The model under review builds one solid part; all positions refer to its coordinate system, in mm. A direction names the side the tool comes from. Round coordinates to 2 decimals unless told otherwise and drop trailing zeros. Loops run counter-clockwise (first coordinate to the right, second up) from the corner with the lowest first, then second, coordinate; pieces in that order, holes last. Notation, with made-up numbers: M 31,65 L 63,65 A9 cw 63,71 Z; hole C 50,89 d5. An arc over 180 degrees is marked long. Return JSON: item names as keys, results as strings. Group by question number.
Q1. Consider section D-D (x = -7). State the section outline as (y, z) points (3 decimals), and give its area (3 significant figures).
Q2. Consider section C-C (y = -1). State the section outline as (x, z) points, and give its area (3 significant figures).
Q3. Draft analysis for pull direction X (two halves, no side actions). For faces 1 (the face through (-12.5, 0, -17)), 2 (the face through (20, 0, 0)), 3 (the face through (10.577, -0.042, 10.636)), state which applies: pulls with the +X half, pulls with the -X half, needs draft (parallel to the pull), parting line crosses it, or undercut.
Q4. To check wall thickness, follow line 1 along Z through (x, y) = (-18, -2.5); line 2 along X through (y, z) = (-15, 6); line 3 along X through (y, z) = (-10, -5.5). State the ranges of each line that lie inside material, in increasing order.
Q5. Clearance check with flat-ended pins moving along their axes: pin 1 Ø2.5 at (x, y) = (17, 3) entering from +Z; pin 2 Ø1.5 at (x, z) = (10, 4.5) entering from +Y; pin 3 Ø1.5 at (x, y) = (7, 1) entering from +Z; pin 4 Ø6 at (y, z) = (-1, -15) entering from -X. State where each tip first meets the part, or that it passes through.
Q6. For faces 4 (the face through (17, 0, 12.5)), 5 (the face through (12.5, 0, -17)), 6 (the face through (-17, 0, 12.5)), list the 3-axis set-ups (+Z, -Z, +X, -X, +Y, -Y) from which the entire face can be reached by the end or side of a thin tool; tool diameter is ignored.
Q7. Consider section A-A (y = -12.5). State the section outline as (x, z) points.
Q8. Consider section B-B (z = -11). Count the separate pieces of the cut face and the enclosed holes in it, and give its area (3 significant figures).
from build123d import *
from OCP.BRepAlgoAPI import BRepAlgoAPI_Cut
from OCP.TopTools import TopTools_ListOfShape

# Parameters (mm, degrees)
CUT_EXTRUDE_2_DEPTH      = 59.108987417
CUT_EXTRUDE_2_DEPTH_BACK = 59.108987417
SKETCH_6_W               = 109.700764472
SKETCH_6_H               = 102.082655829
SKETCH_6_W_2             = 40
SKETCH_6_H_2             = 40
SKETCH_7_W               = 10.430230832
SKETCH_7_H               = 9.900213331
CUT_EXTRUDE_3_DEPTH      = 66.9796091
SKETCH_8_W               = 20.261670598
SKETCH_8_H               = 3
SKETCH_9_W               = 20.800473715
SKETCH_9_H               = 3
SKETCH_11_W              = 20.381404624
SKETCH_11_H              = 3
SKETCH_12_W              = 21.399143843
SKETCH_12_H              = 3


with BuildPart() as part:
    # Sketch 3 → Revolve 1 (revolve)
    with BuildSketch(Plane(origin=(0, 0, 0), x_dir=(0, 0, -1), z_dir=(1, 0, 0))):
        with BuildLine():
            Line((0, 40), (0, -40))
            ThreePointArc((0, -40), (40, 0), (0, 40))
        make_face()
    revolve(axis=Axis((0, 40, 0), (0, -1, 0)))

    # Sketch 4 → Cut-Revolve 3 (revolve, cut)
    with BuildSketch(Plane.XY, mode=Mode.PRIVATE) as cut_revolve_3_sk:
        Polygon((-25, 50), (25, 50), (12.5, 20), (-12.5, 20), align=None)
    revolve(cut_revolve_3_sk.sketch.rotate(Axis((-55.247864245, 0, 0), (1, 0, 0)), 90), axis=Axis((-55.247864245, 0, 0), (1, 0, 0)), mode=Mode.SUBTRACT)


with BuildPart() as cut_revolve_4_tool:
    # Sketch 5 → Cut-Revolve 4 (revolve)
    with BuildSketch(Plane(origin=(0, 0, 0), x_dir=(1, 0, 0), z_dir=(0, 1, 0))):
        Polygon((-50, 25), (-50, -25), (-20, -12.5), (-20, 12.5), align=None)
    revolve(axis=Axis((0, 0, -44.002313129), (0, 0, 1)))


with BuildPart() as part_1:
    add(part.part)

    # Cut-Revolve 4: cut by cut_revolve_4_tool, with a tolerance
    cut_revolve_4_stock = TopTools_ListOfShape()
    cut_revolve_4_stock.Append(part_1.part.wrapped)
    cut_revolve_4_tools = TopTools_ListOfShape()
    cut_revolve_4_tools.Append(cut_revolve_4_tool.part.wrapped)
    cut_revolve_4_cut = BRepAlgoAPI_Cut()
    cut_revolve_4_cut.SetArguments(cut_revolve_4_stock)
    cut_revolve_4_cut.SetTools(cut_revolve_4_tools)
    cut_revolve_4_cut.SetFuzzyValue(0.00001)
    cut_revolve_4_cut.Build()
    add(Compound.cast(cut_revolve_4_cut.Shape()).solids(), mode=Mode.REPLACE)

    # Sketch 6 → Cut-Extrude 2 (cut, two sides: drawn at the far end of the back side and taken through both)
    with BuildSketch(Plane(origin=(0, 0, 0), x_dir=(1, 0, 0), z_dir=(0, 1, 0)).offset(-CUT_EXTRUDE_2_DEPTH_BACK)):
        with Locations((-5.024851986, -5.217653308)):
            Rectangle(SKETCH_6_W, SKETCH_6_H)
        Rectangle(SKETCH_6_W_2, SKETCH_6_H_2, mode=Mode.SUBTRACT)
    extrude(amount=CUT_EXTRUDE_2_DEPTH + CUT_EXTRUDE_2_DEPTH_BACK, mode=Mode.SUBTRACT)

    # Sketch 7 → Cut-Extrude 3 (cut, through all)
    with BuildSketch(Plane(origin=(0, 29.80481839, 0), x_dir=(1, 0, 0), z_dir=(0, 1, 0))):
        Polygon((-12.5, 20), (-12.5, 12.5), (-20, 12.5), (-20, 22.400213331), (-12.5, 22.400213331), align=None)
        with Locations((17.715115416, 17.450106666)):
            Rectangle(SKETCH_7_W, SKETCH_7_H)
        Polygon((-12.5, -12.5), (-12.5, -22.2886307), (-23.264978728, -21.674926225), (-21.87019583, -13.864142), (-20, -12.5), align=None)
        Polygon((12.5, -12.5), (12.5, -20), (16.291064241, -21.981778462), (20, -20), (23.264978728, -15.681813192), (21.632489364, -12.626578567), (20, -12.5), align=None)
    extrude(amount=-CUT_EXTRUDE_3_DEPTH, mode=Mode.SUBTRACT)

    # Sketch 8 → Cut-Revolve 5 (revolve, cut)
    with BuildSketch(Plane(origin=(0, 0, 0), x_dir=(-0.7071067811865477, 0, -0.7071067811865475), z_dir=(0.7071067811865475, 0, -0.7071067811865477)), mode=Mode.PRIVATE) as cut_revolve_5_sk:
        with Locations((25.130835299, 1.5)):
            Rectangle(SKETCH_8_W, SKETCH_8_H)
    revolve(cut_revolve_5_sk.sketch.rotate(Axis((17.737263362, 0, 17.737263362), (-0.7071067811865476, 0, -0.7071067811865475)), 90), axis=Axis((17.737263362, 0, 17.737263362), (-0.7071067811865476, 0, -0.7071067811865475)), mode=Mode.SUBTRACT)

    # Sketch 9 → Cut-Revolve 6 (revolve, cut)
    with BuildSketch(Plane(origin=(0, 0, 0), x_dir=(-0.7071067811865477, 0, 0.7071067811865475), z_dir=(-0.7071067811865475, 0, -0.7071067811865477)), mode=Mode.PRIVATE) as cut_revolve_6_sk:
        with Locations((-25.400236858, 1.5)):
            Rectangle(SKETCH_9_W, SKETCH_9_H)
    revolve(cut_revolve_6_sk.sketch.rotate(Axis((17.65259862, 0, -17.65259862), (-0.7071067811865477, 0, 0.7071067811865475)), 90), axis=Axis((17.65259862, 0, -17.65259862), (-0.7071067811865477, 0, 0.7071067811865475)), mode=Mode.SUBTRACT)

    # Sketch 11 → Cut-Revolve 10 (revolve, cut)
    with BuildSketch(Plane(origin=(0, 0, 0), x_dir=(0.7071067811865476, 0, -0.7071067811865475), z_dir=(0.7071067811865475, 0, 0.7071067811865476)), mode=Mode.PRIVATE) as cut_revolve_10_sk:
        with Locations((-25.190702312, 1.5)):
            Rectangle(SKETCH_11_W, SKETCH_11_H)
    revolve(cut_revolve_10_sk.sketch.rotate(Axis((-18.922569744, 0, 18.922569744), (0.7071067811865476, 0, -0.7071067811865475)), 90), axis=Axis((-18.922569744, 0, 18.922569744), (0.7071067811865476, 0, -0.7071067811865475)), mode=Mode.SUBTRACT)

    # Sketch 12 → Cut-Revolve 11 (revolve, cut)
    with BuildSketch(Plane(origin=(0, 0, 0), x_dir=(0.7071067811865477, 0, 0.7071067811865475), z_dir=(-0.7071067811865475, 0, 0.7071067811865477)), mode=Mode.PRIVATE) as cut_revolve_11_sk:
        with Locations((25.699571922, 1.5)):
            Rectangle(SKETCH_12_W, SKETCH_12_H)
    revolve(cut_revolve_11_sk.sketch.rotate(Axis((0, 0, 0), (0.7071067811865477, 0, 0.7071067811865475)), 90), axis=Axis((0, 0, 0), (0.7071067811865477, 0, 0.7071067811865475)), mode=Mode.SUBTRACT)


solid = part_1.part
Values:
{
 "1": {"outline": "M -18.735,-7 A20 ccw 18.735,-7 L 18.735,7 A20 ccw -18.735,7 Z", "area": "1,230 mm2"},
 "2": {"outline": "M -19.97,-12.5 L -16.5,-12.5 L -12.61,-8.61 L -8.61,-12.61 L -12.5,-16.5 L -12.5,-19.97 L 12.5,-19.97 L 12.5,-16.5 L 8.61,-12.61 L 12.61,-8.61 L 16.5,-12.5 L 19.97,-12.5 L 19.97,12.5 L 16.5,12.5 L 12.61,8.61 L 8.61,12.61 L 12.5,16.5 L 12.5,19.97 L -12.5,19.97 L -12.5,16.5 L -8.61,12.61 L -12.61,8.61 L -16.5,12.5 L -19.97,12.5 Z", "area": "1,280 mm2"},
 "3": {"face 1": "pulls with the -X half", "face 2": "pulls with the +X half", "face 3": "undercut"},
 "4": {"line 1": "z = -12.5 to 12.5", "line 2": "x = -13.23 to 13.23", "line 3": "x = -17.32 to 17.32"},
 "5": {"pin 1": "stops at z = 12.5", "pin 2": "stops at y = 17.73", "pin 3": "stops at z = 20", "pin 4": "stops at x = -20"},
 "6": {"face 4": "+Z, +X, +Y, -Y", "face 5": "-Z, +X, +Y, -Y", "face 6": "+Z, -X, +Y, -Y"},
 "7": {"outline": "M -15.61,-12.5 L -12.5,-12.5 L -12.5,-15.61 L 12.5,-15.61 L 12.5,-12.5 L 15.61,-12.5 L 15.61,12.5 L 12.5,12.5 L 12.5,15.61 L -12.5,15.61 L -12.5,12.5 L -15.61,12.5 Z"},
 "8": {"separate pieces": "1", "enclosed holes": "2", "area": "1,110 mm2"}
}
